The model under review builds one solid part; all positions refer to its coordinate system, in mm. Face numbers are marked on the shaded views. A direction names the side the tool comes from. Coordinates: 2 decimals unless noted, no trailing zeros. Write each loop counter-clockwise with the first axis right and the second up, starting at its lowest first coordinate (ties: lowest second). Pieces come first, ordered by that corner, then holes. Notation, with made-up numbers: M -18.5,34 L -3.5,34 A7 cw -3.5,40 Z; hole C 71.25,26 d4. An arc over 180 degrees is marked long. Answer as a JSON object with one key per item and string values.
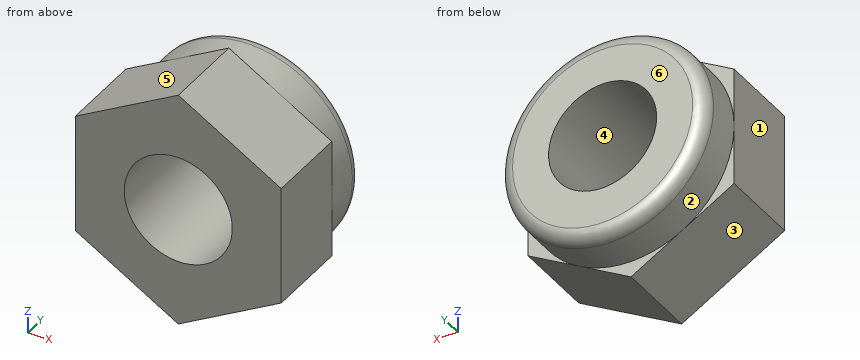
```python
from build123d import *

# Parameters (mm, degrees)
EXTRUDE_1_DEPTH    = 3.2
SKETCH_2_R         = 4
EXTRUDE_2_DEPTH    = 1.8
FILLET_1_R         = 0.5
HOLE_WIZARD_M5_1_D = 4.2


with BuildPart() as part:
    # 草图1 → 凸台-拉伸1 (new body)
    with BuildSketch(Plane(origin=(0, 0, 0), x_dir=(1, 0, 0), z_dir=(0, 1, 0))):
        Polygon((0, 4.618802154), (-4, 2.309401077), (-4, -2.309401077), (0, -4.618802154), (4, -2.309401077), (4, 2.309401077), align=None)
    extrude(amount=EXTRUDE_1_DEPTH)

    # 草图2 → 凸台-拉伸2 (add)
    with BuildSketch(Plane(origin=(0, 3.2, 0), x_dir=(1, 0, 0), z_dir=(0, 1, 0))):
        with Locations(Location((0, 0, 0), (0, 0, 60))):
            Circle(SKETCH_2_R)
    extrude(amount=EXTRUDE_2_DEPTH)

    # 圆角1
    fillet_1_edges = [part.edges().sort_by_distance(p)[0] for p in [
        (-2, 5, 3.464101615),
    ]]
    fillet(fillet_1_edges, radius=FILLET_1_R)

    # M5 螺纹孔1 (through all)
    with Locations(Plane(origin=(0, 5, 0), x_dir=(1, 0, 0), z_dir=(0, 1, 0))):
        with Locations((0, 0)):
            Hole(HOLE_WIZARD_M5_1_D / 2)


solid = part.part
```
(1) For the marked faces 1 and 2, list the 3-axis set-ups (+Z, -Z, +X, -X, +Y, -Y) from which the entire face can be reached by the end or side of a thin tool; tool diameter is ignored.
Results list:
{"face 1": "+Z, -Z, -X, +Y, -Y", "face 2": "+Y"}
(2) Add section B-B on y = 3.6. Give the boundary of the cut face in (x, z).
Results list:
{"outline": "C 0,0 d8; hole C 0,0 d4.2"}
(3) Draft analysis for pull direction Z (two halves, no side actions). For the marked faces 3, 4, 5 and 6, state which applies: released by +Z, released by -Z, zero draft, split by the parting line, or undercut.
Results list:
{"face 3": "released by -Z", "face 4": "undercut", "face 5": "released by +Z", "face 6": "zero draft"}
(4) Wall thickness on line 1 along Z through (x, y) = (0, 3.75); line 2 along Y through (x, z) = (-3.5, -2); line 3 along X through (y, z) = (4.25, -1.25): over which ranges is each line inside the solid? List them lowest first. Write a range as from..to.
Results list:
{"line 1": "-4..-2.1, 2.1..4", "line 2": "0..3.2", "line 3": "-3.8..-1.69, 1.69..3.8"}
(5) For pin 1 Ø0.9 at (x, z) = (0.5, 4) entering from +Y, flat-tipped, find the tip position at first contact; note if it passes through.
Results list:
{"pin 1": "y = 4.99"}
(6) Add section A-A on y = 2.1. Give the boundary of the cut face in (x, z).
Results list:
{"outline": "M -4,-2.31 L 0,-4.62 L 4,-2.31 L 4,2.31 L 0,4.62 L -4,2.31 Z; hole C 0,0 d4.2"}
